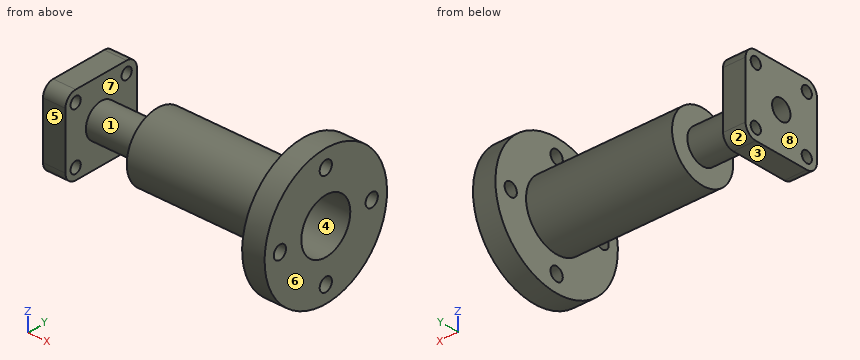
from build123d import *

# Parameters (mm, degrees)
SKETCH2_W              = 70
SKETCH2_H              = 70
SKETCH2_R              = 5
SKETCH2_R_2            = 9
BOSS_EXTRUDE1_DEPTH    = 20
FILLET1_R              = 10
F_12_0MM_DOWEL_HOLE1_D = 12


with BuildPart() as part:
    # Sketch1 → Revolve1 (revolve)
    with BuildSketch(Plane.XY, mode=Mode.PRIVATE) as revolve1_sk:
        Polygon((200, 24), (200, 60), (180, 60), (180, 30), (50, 30), (50, 15), (0, 15), (0, 9), (56, 9), (56, 24), align=None)
    revolve(revolve1_sk.sketch.rotate(Axis((0, 0, 0), (1, 0, 0)), 90), axis=Axis((0, 0, 0), (1, 0, 0)))

    # Sketch2 → Boss-Extrude1 (add)
    with BuildSketch(Plane.ZY):
        Rectangle(SKETCH2_W, SKETCH2_H)
        with Locations((-25, 25)):
            Circle(SKETCH2_R, mode=Mode.SUBTRACT)
        with Locations((25, 25)):
            Circle(SKETCH2_R, mode=Mode.SUBTRACT)
        with Locations(Location((25, -25, 0), (0, 0, 180))):
            Circle(SKETCH2_R, mode=Mode.SUBTRACT)
        with Locations(Location((-25, -25, 0), (0, 0, 180))):
            Circle(SKETCH2_R, mode=Mode.SUBTRACT)
        Circle(SKETCH2_R_2, mode=Mode.SUBTRACT)
    extrude(amount=BOSS_EXTRUDE1_DEPTH)

    # Fillet1
    fillet1_edges = [part.edges().sort_by_distance(p)[0] for p in [
        (-10, -35, 35),
        (-10, 35, 35),
        (-10, 35, -35),
        (-10, -35, -35),
    ]]
    fillet(fillet1_edges, radius=FILLET1_R)

    # Ø12.0mm Dowel Hole1 (through all)
    with Locations(Plane(origin=(200, 0, 0), x_dir=(0, 0, -1), z_dir=(1, 0, 0))):
        with Locations((45, 0), (0, 45), (-45, 0), (0, -45)):
            Hole(F_12_0MM_DOWEL_HOLE1_D / 2)


solid = part.part
Model file for the job. Use its own axes, mm. Face numbers are marked on the shaded views. A direction names the side the tool comes from. Give positions to 0.01 mm unless a question says otherwise; leave off trailing zeros. Order: outer loops, then holes, each group sorted by start corner. A loop starts at its lowest first (then second) coordinate and runs counter-clockwise, first axis right, second up. Notation, with made-up numbers: (11.25, -25) - (15.25, -25) arc R29 cw to (15.25, 13) - close; hole circle Ø11 at (-12, -5.75). An arc over 180 degrees is marked (long way). Write item = value, one per line. Start each with the question number.
1. Cut at C-C, the plane y = -48.5. List the corners of the cut face in (x, z).
2. Probe line 1 along Z through (x, y) = (-11, -25); line 2 along Y through (x, z) = (191.25, 0); line 3 along Z through (x, y) = (102, -1). List the from-to ranges inside material, lowest first.
3. Cut at A-A, the plane y = 0. State how many separate pieces and enclosed holes the cut face has, and give its area (3 significant figures).
4. Cut at D-D, the plane x = 88.5. List the corners of the cut face in (y, z).
5. Drop flat-ended pins along their axis: P1, Ø5, axis at y = -2.5, z = -7.5, coming from the +X side; P2, Ø14.5, axis at y = 0, z = 0, coming from the +X side; P3, Ø22, axis at x = -15, y = 2, coming from the -Z side; P4, Ø4, axis at x = 49, z = -5.5, coming from the -Y side. Give the stop position or say it passes through.
6. Two-plate mould, pull along X, no slides. Class the marked faces 5, 6, 7 and 8: pulls with the +X half, pulls with the -X half, needs draft (parallel to the pull), parting line crosses it, or undercut.
7. Which spindle directions (+Z, -Z, +X, -X, +Y, -Y) get a long thin tool onto all of the face, cutting with end or side? Do the marked faces 1, 2, 3 and 4. Say none if no direction does.
Taken from the geometry:
q1.outline = (180, -35.32) - (200, -35.32) - (200, -4.87) - (180, -4.87) - close; (180, 4.87) - (200, 4.87) - (200, 35.32) - (180, 35.32) - close
q2.line_1 = -35 to -30, -20 to 20, 30 to 35
q2.line_2 = -60 to -51, -39 to -24, 24 to 39, 51 to 60
q2.line_3 = -29.98 to -23.98, 23.98 to 29.98
q3.separate_pieces = 4
q3.enclosed_holes = 0
q3.area = 4,340 mm²
q4.outline = circle Ø60 at (0, 0); hole circle Ø48 at (0, 0)
q5.P1 = 56
q5.P2 = through
q5.P3 = -35
q5.P4 = -29.76
q6.face_5 = needs draft
q6.face_6 = pulls with the +X half
q6.face_7 = undercut
q6.face_8 = pulls with the -X half
q7.face_1 = none
q7.face_2 = -Z, -X, +Y
q7.face_3 = -Z, -X, +Y, -Y
q7.face_4 = +X
